from build123d import *

# Parameters (mm, degrees)
SKETCH1_W           = 41.509557428
SKETCH1_H           = 20.45985577
SKETCH1_R           = 3
SKETCH1_R_2         = 3.3
SKETCH1_R_3         = 1.725
BOSS_EXTRUDE1_DEPTH = 10
SKETCH2_R           = 7.6
BOSS_EXTRUDE2_DEPTH = 7
SKETCH3_R           = 2.525
CUT_EXTRUDE1_DEPTH  = 43.062691409


with BuildPart() as part:
    # Sketch1 → Boss-Extrude1 (new body)
    with BuildSketch(Plane(origin=(0, 0, 0), x_dir=(1, 0, 0), z_dir=(0, 1, 0))):
        with Locations((14.647059063, -4.835923918)):
            Rectangle(SKETCH1_W, SKETCH1_H)
        with Locations(Location((-0.01006999, -10.957446633, 0), (0, 0, 270))):
            Circle(SKETCH1_R, mode=Mode.SUBTRACT)
        with Locations(Location((10.060612969, 0, 0), (0, 0, 270))):
            Circle(SKETCH1_R_2, mode=Mode.SUBTRACT)
        with Locations(Location((10.060612969, -10.957446633, 0), (0, 0, 270))):
            Circle(SKETCH1_R_3, mode=Mode.SUBTRACT)
        Polygon((2.480175999, 1.419939088), (0.010384677, 2.857864965), (-2.469791322, 1.437925877), (-2.480175999, -1.419939088), (-0.010384677, -2.857864965), (2.469791322, -1.437925877), align=None, mode=Mode.SUBTRACT)
    extrude(amount=BOSS_EXTRUDE1_DEPTH)

    # Sketch2 → Boss-Extrude2 (add)
    with BuildSketch(Plane(origin=(0, 10, 0), x_dir=(1, 0, 0), z_dir=(0, 1, 0))):
        with Locations(Location((23.760138251, -4.917169795, 0), (0, 0, 270))):
            Circle(SKETCH2_R)
    extrude(amount=BOSS_EXTRUDE2_DEPTH)

    # Sketch3 → Cut-Extrude1 (cut, through all)
    with BuildSketch(Plane(origin=(0, 17, 0), x_dir=(1, 0, 0), z_dir=(0, 1, 0))):
        with Locations(Location((23.760138251, -4.917169795, 0), (0, 0, 270))):
            Circle(SKETCH3_R)
    extrude(amount=-CUT_EXTRUDE1_DEPTH, mode=Mode.SUBTRACT)


solid = part.part
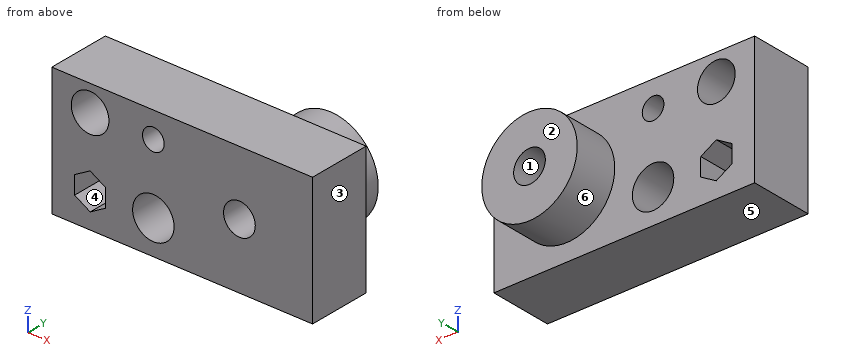
Build history of the part. All positions in model axes, mm. Face numbers are marked on the shaded views. A direction names the side the tool comes from. Give positions to 0.01 mm unless a question says otherwise; leave off trailing zeros. Write each loop counter-clockwise with the first axis right and the second up, starting at its lowest first coordinate (ties: lowest second). Pieces come first, ordered by that corner, then holes. Notation, with made-up numbers: (76, -37.5) - (90, -37.5) arc R30 cw to (90, 1.5) - close; hole circle Ø11 at (-35, 58.5). An arc over 180 degrees is marked (long way). Use one line per item in the form item = value. Start each with the question number.
1. Probe line 1 (X direction, y = 3.75, z = 12.25); line 2 (X direction, y = 7.5, z = 12); line 3 (Y direction, x = 15, z = -2.5). List the from-to ranges inside material, lowest first. Write a range as [from, to].
2. Band-saw the part on A-A on x = 1. Write the cut outline in (y, z), plus the area to 3 significant figures.
3. Band-saw the part on D-D on y = 13.5. Write the cut outline in (x, z) (3 decimals).
4. Band-saw the part on C-C on z = 0. Write the cut outline in (x, y).
5. Drop a flat-ended pin along its axis: pin 1 Ø8.5 at (x, z) = (10.06, 0) entering from +Y. Give the stop position or say it passes through.
6. Band-saw the part on B-B on y = 1.5. Write the cut outline in (x, z) (3 decimals).
7. Two-plate mould, pull along X, no slides. Class the marked faces 1, 2 and 3: released by +X, released by -X, zero draft, split by the parting line, or undercut.
8. 3-axis set-ups, long thin cutter, end or side, ignore diameter. For the marked faces 4, 5 and 6: which of +Z, -Z, +X, -X, +Y, -Y reach the whole face in a straight line?
Conclusion:
q1.line_1 = [-6.11, -2.72], [2.7, 8.92], [11.2, 35.4]
q1.line_2 = [-6.11, -2.82], [2.8, 8.69], [11.43, 35.4]
q1.line_3 = [0, 10]
q2.outline = (0, -5.39) - (10, -5.39) - (10, -2.28) - (0, -2.28) - close; (0, 2.28) - (10, 2.28) - (10, 8.13) - (0, 8.13) - close; (0, 13.78) - (10, 13.78) - (10, 15.07) - (0, 15.07) - close
q2.area = 102 mm²
q3.outline = circle Ø15.2 at (23.76, 4.917); hole circle Ø5.05 at (23.76, 4.917)
q4.outline = (-6.11, 0) - (-2.48, 0) - (-2.48, 10) - (-6.11, 10) - close; (2.48, 0) - (6.76, 0) - (6.76, 10) - (2.48, 10) - close; (13.36, 0) - (35.4, 0) - (35.4, 10) - (29.56, 10) - (29.56, 17) - (17.97, 17) - (17.97, 10) - (13.36, 10) - close
q5.pin_1 = 10
q6.outline = (-6.108, -5.394) - (35.402, -5.394) - (35.402, 15.066) - (-6.108, 15.066) - close; hole circle Ø6 at (-0.01, 10.957); hole (-2.48, 1.42) - (-2.47, -1.438) - (0.01, -2.858) - (2.48, -1.42) - (2.47, 1.438) - (-0.01, 2.858) - close; hole circle Ø6.6 at (10.061, 0); hole circle Ø3.45 at (10.061, 10.957); hole circle Ø5.05 at (23.76, 4.917)
q7.face_1 = undercut
q7.face_2 = zero draft
q7.face_3 = released by +X
q8.face_4 = +Y, -Y
q8.face_5 = -Z, +X, -X, +Y, -Y
q8.face_6 = +Y
